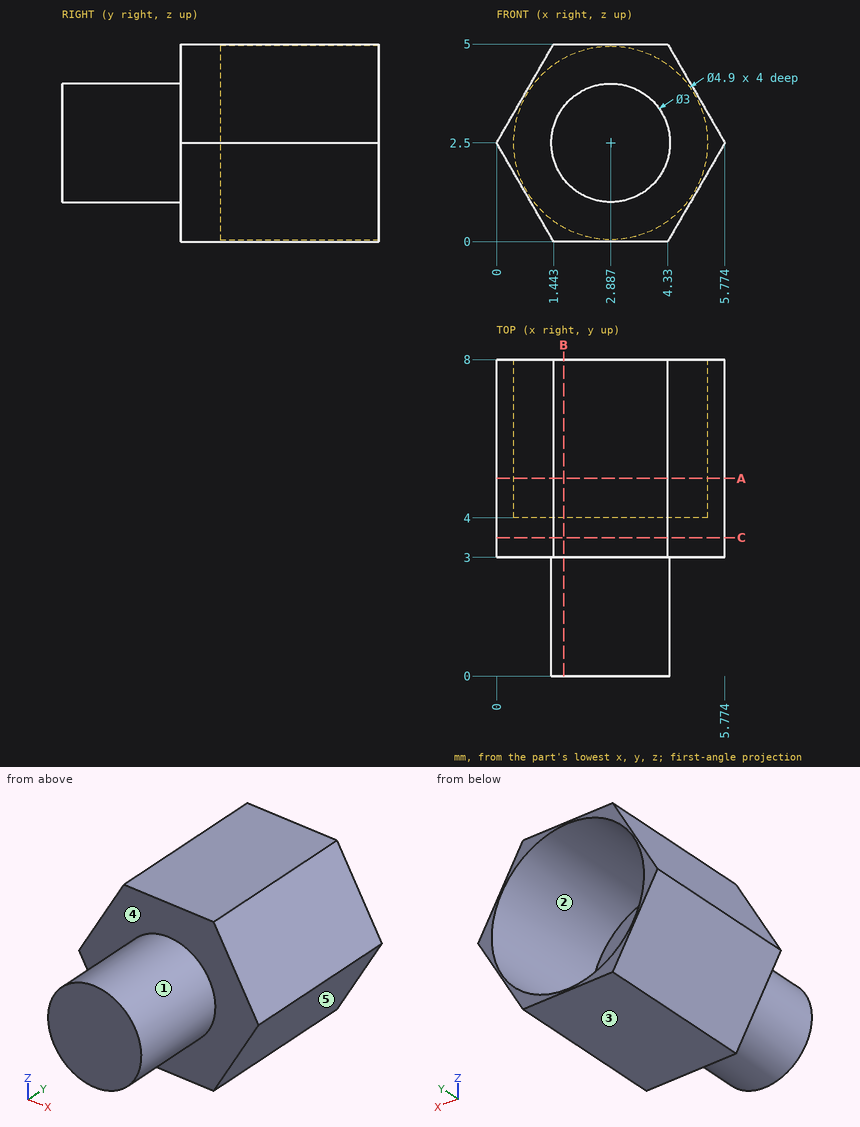
Input: dimensioned drawing with shaded views. Units: mm. Origin: part minimum x, y, z. A direction names the side the tool comes from. Coordinates: 2 decimals unless noted, no trailing zeros. Loops run counter-clockwise (first coordinate to the right, second up) from the corner with the lowest first, then second, coordinate; pieces in that order, holes last.
Q1. Set-up query: the marked faces 4 and 5. Return all of +Z, -Z, +X, -X, +Y, -Y with unobstructed straight access to the full face (end or side cutting, diameter ignored); none if empty.
Results are:
face 4: -Y
face 5: -Z, +X, +Y, -Y
Q2. Section A-A, the plane y = 5. Return the cut outline in (x, z).
Results are:
outline: (0, 2.5) - (1.44, 0) - (4.33, 0) - (5.77, 2.5) - (4.33, 5) - (1.44, 5) - close; hole circle Ø4.9 at (2.89, 2.5)
Q3. Section B-B, the plane x = 1.7. Return the cut outline in (y, z).
Results are:
outline: (0, 1.58) - (3, 1.58) - (3, 0) - (8, 0) - (8, 0.36) - (4, 0.36) - (4, 4.64) - (8, 4.64) - (8, 5) - (3, 5) - (3, 3.42) - (0, 3.42) - close
Q4. Line query: line 1 along Y through (x, z) = (1.4, 3.1); line 2 along Y through (x, z) = (1.75, 2.5); line 3 along X through (y, z) = (5.5, 2.35) (1 decimal). Output: solid intervals per line, ascending.
Results are:
line 1: y = 3 to 4
line 2: y = 0 to 4
line 3: x = 0.1 to 0.4, 5.3 to 5.7
Q5. Section C-C, the plane y = 3.5. Return the cut outline in (x, z).
Results are:
outline: (0, 2.5) - (1.44, 0) - (4.33, 0) - (5.77, 2.5) - (4.33, 5) - (1.44, 5) - close
Q6. Mould query, pull axis X, two halves, no side actions, for the marked faces 1, 2 and 3. Classes: +X half, -X half, draft (parallel to the pull), parting line (faces both ways), or undercut.
Results are:
face 1: parting line
face 2: undercut
face 3: draft
Q7. Contact query for flat-ended pins moving along their axis: pin 1 (1.5 mm diameter, centred on x = 3, y = 2, fed in from +Z); pin 2 (1 mm diameter, centred on x = 2, z = 1.5, fed in from +Y). Output: stop coordinate, or through.
Results are:
pin 1: stops at z = 4
pin 2: stops at y = 4
